Check sheet for the drawn part. Datum: minimum x, y, z corner. Units: mm. A direction names the side the tool comes from. Coordinates: 2 decimals unless noted, no trailing zeros. Order: outer loops, then holes, each group sorted by start corner. A loop starts at its lowest first (then second) coordinate and runs counter-clockwise, first axis right, second up. Notation, with made-up numbers: M -16.5,43 L 9.5,43 A29 cw 9.5,68 Z; hole C 87,-37.75 d9. An arc over 180 degrees is marked long. Answer in a Markdown table with one row per item. Add a question column.
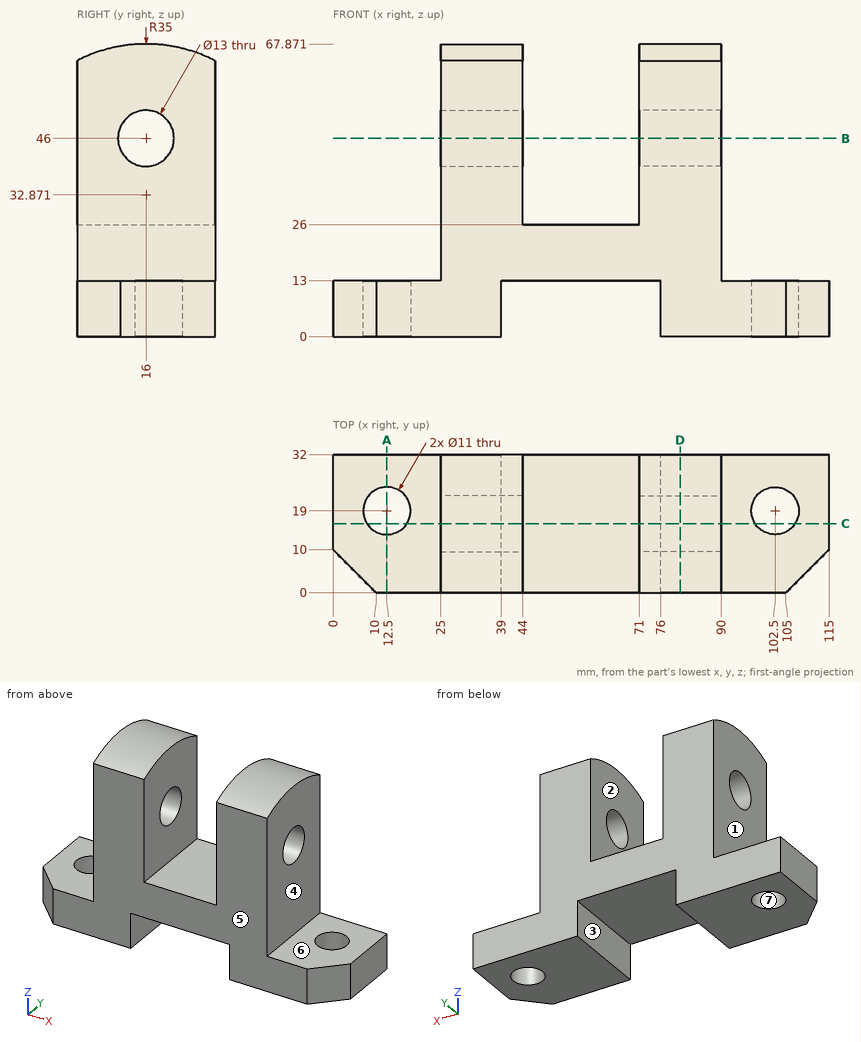
1. Section check C-C on y = 16. State how many separate pieces and enclosed holes the cut face has, then the cut area to 3 significant figures.
2. Release check for a two-part mould opening along Y. For the marked faces 5, 6 and 7 record: released by +Y, released by -Y, zero draft, split by the parting line, or undercut.
3. Go/stop test with flat-tipped pins: pin 1 Ø9.5 at (y, z) = (10, 44) entering from +X; pin 2 Ø12.5 at (x, y) = (12, 22) entering from +Z; pin 3 Ø9.5 at (x, y) = (59, 23) entering from -Z. Record where each tip stops, or that it passes through.
4. Section check B-B on z = 46. Enter the section's corners in (x, y), then the cut area to 3 significant figures.
5. Section check A-A on x = 12.5. Enter the section's corners in (y, z).
6. Section check D-D on x = 80.5. Enter the section's corners in (y, z), then the cut area to 3 significant figures.
7. Set-up check for the marked faces 1, 2, 3 and 4: record each of +Z, -Z, +X, -X, +Y, -Y from which the full face is reachable in a straight line by a thin tool's end or side.
8. Scan lines: line 1 (Y direction, x = 102.5, z = 10); line 2 (X direction, y = 22.5, z = 5); line 3 (X direction, y = 23, z = 25). Record each from-to range of solid material in increasing order.
Result sheet:
| question | item | result |
|---|---|---|
| 1 | separate pieces | 5 |
| 1 | enclosed holes | 0 |
| 1 | area | 2,720 mm^2 |
| 2 | face 5 | released by -Y |
| 2 | face 6 | zero draft |
| 2 | face 7 | undercut |
| 3 | pin 1 | x = 90 |
| 3 | pin 2 | z = 13 |
| 3 | pin 3 | z = 13 |
| 4 | outline | M 25,0 L 44,0 L 44,9.5 L 25,9.5 Z; M 25,22.5 L 44,22.5 L 44,32 L 25,32 Z; M 71,0 L 90,0 L 90,9.5 L 71,9.5 Z; M 71,22.5 L 90,22.5 L 90,32 L 71,32 Z |
| 4 | area | 722 mm^2 |
| 5 | outline | M 0,0 L 13.5,0 L 13.5,13 L 0,13 Z; M 24.5,0 L 32,0 L 32,13 L 24.5,13 Z |
| 6 | outline | M 0,0 L 32,0 L 32,64 A35 ccw 0,64 Z; hole C 16,46 d13 |
| 6 | area | 2,000 mm^2 |
| 7 | face 1 | +Z, -X, +Y, -Y |
| 7 | face 2 | +Z, +Y, -Y |
| 7 | face 3 | -Z, +Y, -Y |
| 7 | face 4 | +Z, +X, +Y, -Y |
| 8 | line 1 | 0 to 13.5, 24.5 to 32 |
| 8 | line 2 | 0 to 8.26, 16.74 to 39, 76 to 98.26, 106.74 to 115 |
| 8 | line 3 | 25 to 90 |
